Autodesk Inventor part; units mm, degrees
ref_plane "YZ Plane" through (0, 0, 0) normal (1, 0, 0) x (0, 1, 0)
ref_plane "XZ Plane" through (0, 0, 0) normal (0, 1, 0) x (-1, 0, 0)
ref_plane "XY Plane" through (0, 0, 0) normal (0, 0, 1) x (1, 0, 0)
sketch "Sketch1" plane through (0, 0, 0) normal (0, 1, 0) x (-1, 0, 0)
  line L0 (-15.875, 15.875) -> (15.875, 15.875)
  line L1 (15.875, 15.875) -> (15.875, -15.875)
  line L2 (15.875, -15.875) -> (-15.875, -15.875)
  line L3 (-15.875, -15.875) -> (-15.875, 15.875)
  line L4 (-15.875, 15.875) -> (15.875, -15.875) construction
  line L5 (15.875, 15.875) -> (-15.875, -15.875) construction
  point P0 (0, 0)
  dimension "width" = 31.75
  dimension "depth" = 31.75
extrude "Extrusion1" add sketch "Sketch1" against normal blind 38.1
sketch "Sketch2" plane through (15.875, 0, 15.875) normal (1, 0, 0) x (0, 0, -1)
  line L0 (0, -38.1) -> (31.75, -38.1)
  line L1 (31.75, -38.1) -> (12.7, -38.1)
  line L2 (12.7, -38.1) -> (12.7, -5.08)
  line L3 (12.7, -5.08) -> (31.75, -5.08)
  line L4 (31.75, -5.08) -> (31.75, -38.1)
  point P0 (15.875, 0)
  dimension "dLinkHeight" = 33.02
  dimension "dLinkWidth" = 19.05
extrude "Extrusion2" cut sketch "Sketch2" against normal blind 19.05
sketch "Sketch6" plane through (0, 0, 0) normal (0, 1, 0) x (1, 0, 0)
  line L0 (15.875, 15.875) -> (15.875, -15.875) construction
  line L1 (15.875, -9.525) -> (-15.875, -9.525) construction
  line L2 (-15.875, -15.875) -> (-15.875, 15.875) construction
  line L3 (-9.525, -15.875) -> (-9.525, 15.875) construction
  line L4 (-15.875, 15.875) -> (15.875, 15.875) construction
  line L5 (15.875, -15.875) -> (-15.875, -15.875) construction
  circle A0 centre (-9.525, -9.525) radius 4.2164
  point P0 (0, 0)
  dimension "widthCenterLine" = 6.35
  dimension "depthCenterLine" = 6.35
  dimension "diamHeadCapScrew" = 8.4328
extrude "Extrusion3" cut sketch "Sketch6" against normal blind 6.858
sketch "Sketch7" plane through (-9.525, -6.858, 9.525) normal (0, 1, 0) x (1, 0, 0)
  circle A0 centre (0, 0) radius 2.413
  point P0 (9.525, 9.525)
  dimension "capScrewThroughHole" = 4.826
extrude "Extrusion4" cut sketch "Sketch7" against normal through all
fillet "Fillet1" radius 3.175 1 edges at (-3.175, -21.59, 3.175)
fillet "Fillet2" radius 3.175 3 edges at (-2.2451, -5.08, 2.2451) (-3.175, -5.08, -7.9375) (7.9375, -5.08, 3.175)
fillet "Fillet3" radius 3.175 3 edges at (-15.875, -19.05, 15.875) (-15.875, -19.05, -15.875) (15.875, -19.05, 15.875)
equation "\"widthCenterLine\" = -0.5 * dLinkWidth + 0.5 * width"
equation "\"depthCenterLine\" = -0.5 * dLinkWidth + 0.5 * depth"
equation "\"capScrewSpacing\" = 0.508"
equation "\"depthCapScrewSpacing\" = 0.508"
properties part number "cornerBracketForDLink"
Here's how the part is built. I have some questions about the finished solid (model axes, mm). A direction names the side the tool comes from. Coordinates: 2 decimals unless noted, no trailing zeros. Order: outer loops, then holes, each group sorted by start corner. A loop starts at its lowest first (then second) coordinate and runs counter-clockwise, first axis right, second up.
1) Imagine slicing it at A-A on x = 3. List the corners of the cut face in (y, z) for me (3 decimals), and give its area (3 significant figures).
2) Will these pins go through, and if not, where does the flat tip stop? pin 1 (6.5 mm diameter, centred on x = -9.525, z = 9.525, fed in from +Y); pin 2 (17.5 mm diameter, centred on x = 10.5, z = -6.5, fed in from -Y); pin 3 (1 mm diameter, centred on x = 7, y = -19.5, fed in from -Z) (3 decimals); pin 4 (4.5 mm diameter, centred on x = -9.525, z = 9.525, fed in from +Y).
3) Which directions (+Z, -Z, +X, -X, +Y, -Y) give clear straight access to the entire face, cutting with the end or side of a thin tool? Please do faces 1 (the face through (0, 0, 0)), 2 (the face through (-7.71, -6.858, 11.34)), 3 (the face through (8, -23, 3.175)).
4) Imagine slicing it at D-D on z = -4. List the corners of the cut face in (x, y) for me (3 decimals).
5) I need wall thicknesses on line 1 (Z direction, x = 12.5, y = -26) (3 decimals); line 2 (Y direction, x = 6.5, z = -1); line 3 (X direction, y = -19.5, z = -5.5) (3 decimals). Which ranges of each line are inside material? Lowest first, please.
6) Imagine slicing it at C-C on z = 9. List the corners of the cut face in (x, y) for me (3 decimals).
7) We'd pull the mould along X, two halves only. Please class faces 4 (the face through (-12.87, -3.38, 12.09)), 5 (the face through (15.875, -15, 5)), 6 (the face through (-3, -38.1, 4)): +X half, -X half, draft (parallel to the pull), parting line (faces both ways), or undercut.
8) Imagine slicing it at B-B on x = -8. List the corners of the cut face in (y, z) for me (3 decimals).
Response values:
1. outline: (-38.1, 3.175) - (-8.255, 3.175) arc R3.175 cw to (-5.08, 0) - (-5.08, -15.875) - (0, -15.875) - (0, 15.875) - (-38.1, 15.875) - close
1. area: 583 mm2
2. pin 1: stops at y = -6.86
2. pin 2: stops at y = -6.01
2. pin 3: stops at z = 3.175
2. pin 4: passes through
3. face 1: +Z, -Z, +X, -X, +Y
3. face 2: +Y
3. face 3: -Z, +X, -Y
4. outline: (-15.875, -38.1) - (-3.175, -38.1) - (-3.175, -8.255) arc R3.175 cw to (0, -5.08) - (15.875, -5.08) - (15.875, 0) - (-15.875, 0) - close
5. line 1: z = 3.175 to 15.875
5. line 2: y = -5.08 to 0
5. line 3: x = -15.875 to -3.175
6. outline: (-15.875, -38.1) - (-11.88, -38.1) - (-11.88, -6.858) - (-13.709, -6.858) - (-13.709, 0) - (-15.875, 0) - close; (-7.17, -38.1) - (15.875, -38.1) - (15.875, 0) - (-5.341, 0) - (-5.341, -6.858) - (-7.17, -6.858) - close
7. face 4: undercut
7. face 5: +X half
7. face 6: draft
8. outline: (-38.1, -15.875) - (0, -15.875) - (0, 5.594) - (-6.858, 5.594) - (-6.858, 7.655) - (-38.1, 7.655) - close; (-38.1, 11.395) - (-6.858, 11.395) - (-6.858, 13.456) - (0, 13.456) - (0, 15.875) - (-38.1, 15.875) - close
